```python
from build123d import *

# Parameters (mm, degrees)
SKETCH1_W           = 25.4
SKETCH1_H           = 25.4
SKETCH1_W_2         = 19.05
SKETCH1_H_2         = 19.05
BOSS_EXTRUDE1_DEPTH = 355.6
CUT_EXTRUDE1_START  = -25.4
SKETCH2_R           = 3.3734375
CUT_EXTRUDE1_DEPTH  = 25.4
CUT_EXTRUDE2_START  = -25.4
SKETCH3_R           = 3.3734375
CUT_EXTRUDE2_DEPTH  = 25.4


with BuildPart() as part:
    # Sketch1 → Boss-Extrude1 (new body)
    with BuildSketch(Plane(origin=(0, 0, 0), x_dir=(1, 0, 0), z_dir=(0, 1, 0))):
        with Locations((12.7, 12.7)):
            Rectangle(SKETCH1_W, SKETCH1_H)
        with Locations((12.7, 12.7)):
            Rectangle(SKETCH1_W_2, SKETCH1_H_2, mode=Mode.SUBTRACT)
    extrude(amount=BOSS_EXTRUDE1_DEPTH)

    # Sketch2 → Cut-Extrude1 (cut)
    with BuildSketch(Plane(origin=(25.4, 0, 0), x_dir=(0, 0, -1), z_dir=(1, 0, 0)).offset(CUT_EXTRUDE1_START)):
        with Locations((12.7, 12.7)):
            Circle(SKETCH2_R)
        with Locations((12.7, 177.8)):
            Circle(SKETCH2_R)
    extrude(amount=CUT_EXTRUDE1_DEPTH, mode=Mode.SUBTRACT)

    # Sketch3 → Cut-Extrude2 (cut)
    with BuildSketch(Plane.XY.offset(CUT_EXTRUDE2_START)):
        with Locations((12.7, 342.9)):
            Circle(SKETCH3_R)
    extrude(amount=CUT_EXTRUDE2_DEPTH, mode=Mode.SUBTRACT)


solid = part.part
```
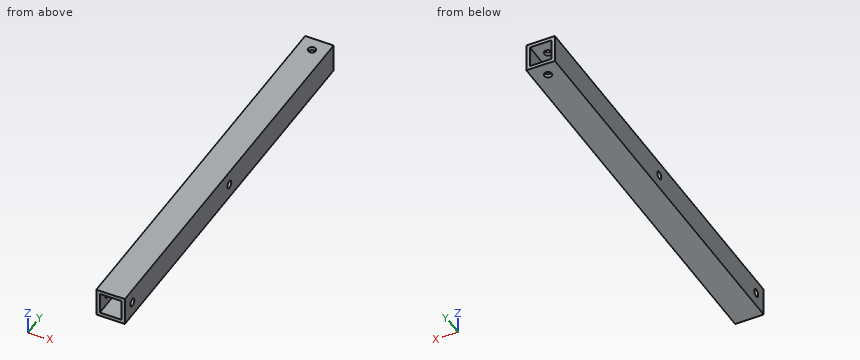
Check sheet for the modelled part. Datum: model origin and axes. Units: mm. Give positions to 0.01 mm unless a question says otherwise; leave off trailing zeros. Write each loop counter-clockwise with the first axis right and the second up, starting at its lowest first coordinate (ties: lowest second). Pieces come first, ordered by that corner, then holes.
Item 1: Scan lines: L1, parallel to Y at x = 1.9, z = -12.7; L2, parallel to Y at x = 12.7, z = -24.5; L3, parallel to Z at x = 13, y = 293 (3 decimals). Record each from-to range of solid material in increasing order.
Item 2: Cross-section at B-B (y = 306). Enter the section's corners in (x, z) (3 decimals).
Item 3: Cross-section at C-C (y = 12.7). Enter the section's corners in (x, z) (3 decimals).
Item 4: Cross-section at A-A (x = 12.7). Enter the section's corners in (y, z) (3 decimals).
Report:
1. L1: y = 0 to 9.33, 16.07 to 174.43, 181.17 to 355.6
1. L2: y = 0 to 339.53, 346.27 to 355.6
1. L3: z = -25.4 to -22.225, -3.175 to 0
2. outline: (0, -25.4) - (25.4, -25.4) - (25.4, 0) - (0, 0) - close; hole (3.175, -22.225) - (22.225, -22.225) - (22.225, -3.175) - (3.175, -3.175) - close
3. outline: (0, -25.4) - (25.4, -25.4) - (25.4, -16.073) - (22.225, -16.073) - (22.225, -22.225) - (3.175, -22.225) - (3.175, -16.073) - (0, -16.073) - close; (0, -9.327) - (3.175, -9.327) - (3.175, -3.175) - (22.225, -3.175) - (22.225, -9.327) - (25.4, -9.327) - (25.4, 0) - (0, 0) - close
4. outline: (0, -25.4) - (339.527, -25.4) - (339.527, -22.225) - (0, -22.225) - close; (0, -3.175) - (339.527, -3.175) - (339.527, 0) - (0, 0) - close; (346.273, -25.4) - (355.6, -25.4) - (355.6, -22.225) - (346.273, -22.225) - close; (346.273, -3.175) - (355.6, -3.175) - (355.6, 0) - (346.273, 0) - close
